Can you work these out from the drawing? Everything is in mm from the part's minimum corner. Round coordinates to 2 decimals unless told otherwise and drop trailing zeros. Loops run counter-clockwise (first coordinate to the right, second up) from the corner with the lowest first, then second, coordinate; pieces in that order, holes last. Notation, with made-up numbers: (-7, -30) - (50, -30) arc R37 ccw to (50, 7) - close; hole circle Ø3 at (6, 68.25). An arc over 180 degrees is marked (long way). Return JSON: item names as keys, results as strings. Group by question number.
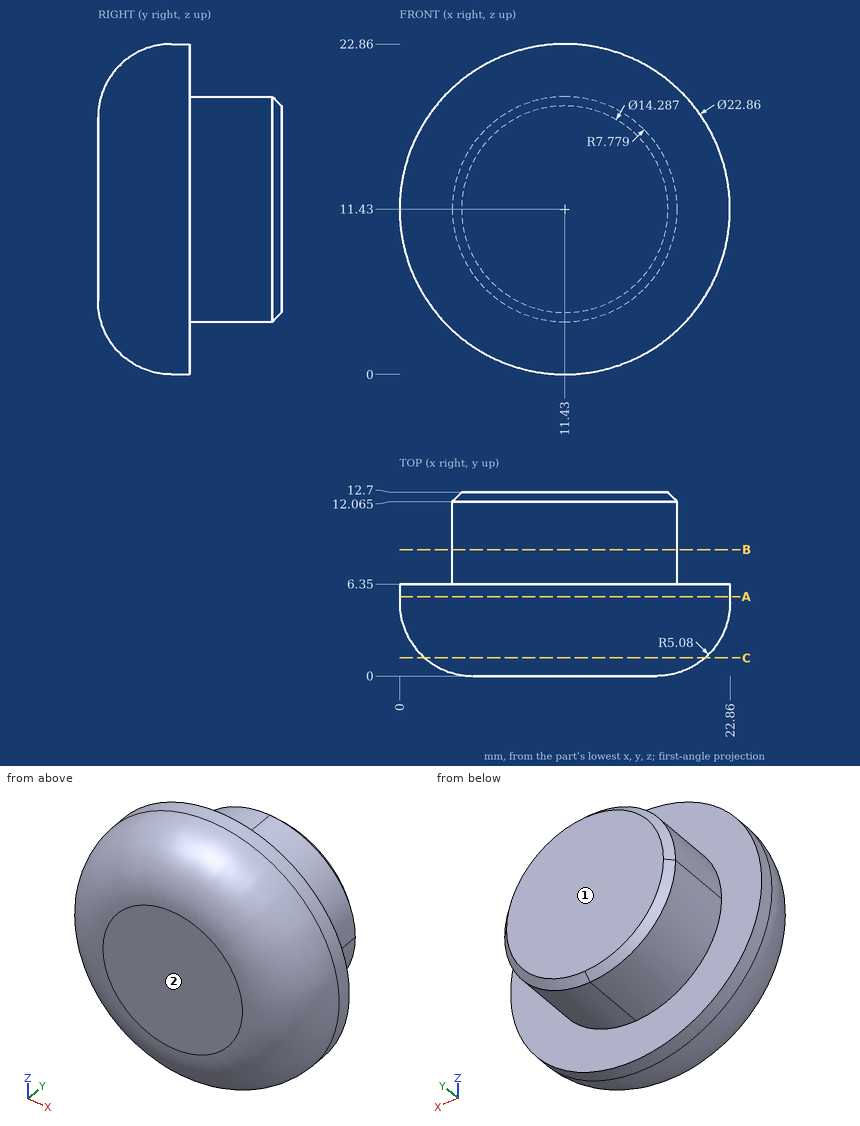
Q1. If we mould it in two halves opening along Y, with no side actions, what happens to the marked faces 1 and 2? For each: +Y half, -Y half, draft (parallel to the pull), parting line (faces both ways), or undercut.
Q2. Please list where these lines run through material, in increasing order: line 1 (X direction, y = 6.5, z = 11.5); line 2 (Z direction, x = 19, y = 3.25) (1 decimal); line 3 (Z direction, x = 17.75, y = 10) (1 decimal).
Q3. Imagine slicing it at A-A, the plane y = 5.5. List the corners of the cut face in (x, z) for me.
Q4. Imagine slicing it at B-B, the plane y = 8.75. List the corners of the cut face in (x, z) for me, and give its area (3 significant figures).
Q5. Will these pins go through, and if not, where does the flat tip stop? pin 1 Ø3 at (x, y) = (14.5, 7.5) entering from +Z (1 decimal); pin 2 Ø1 at (x, y) = (16, 9.5) entering from -Z; pin 3 Ø4 at (x, z) = (3, 18) entering from -Y.
Q6. Imagine slicing it at C-C, the plane y = 1.25. List the corners of the cut face in (x, z) for me (1 decimal).
Output values:
{
 "1": {"face 1": "+Y half", "face 2": "-Y half"},
 "2": {"line 1": "x = 3.65 to 19.21", "line 2": "z = 3.3 to 19.5", "line 3": "z = 6.9 to 16"},
 "3": {"outline": "circle Ø22.86 at (11.43, 11.43)"},
 "4": {"outline": "circle Ø15.56 at (11.43, 11.43)", "area": "190 mm^2"},
 "5": {"pin 1": "stops at z = 22.7", "pin 2": "stops at z = 4.8", "pin 3": "stops at y = 0.57"},
 "6": {"outline": "circle Ø19.4 at (11.4, 11.4)"}
}
